Check sheet for the modelled part. Datum: model origin and axes. Units: mm. Round coordinates to 2 decimals unless told otherwise and drop trailing zeros. Loops run counter-clockwise (first coordinate to the right, second up) from the corner with the lowest first, then second, coordinate; pieces in that order, holes last. Notation, with made-up numbers: (-38, 25.5) - (7, 25.5) arc R14 ccw to (7, 43.5) - close; hole circle Ø8 at (50, -5.75). An arc over 180 degrees is marked (long way). Return JSON: item names as keys, results as strings.
Autodesk Inventor part; units mm, degrees
ref_plane "YZ Plane" through (0, 0, 0) normal (1, 0, 0) x (0, 1, 0)
ref_plane "XZ Plane" through (0, 0, 0) normal (0, 1, 0) x (-1, 0, 0)
ref_plane "XY Plane" through (0, 0, 0) normal (0, 0, 1) x (1, 0, 0)
sketch "Sketch1" plane through (0, 0, 0) normal (0, 0, 1) x (1, 0, 0)
  line L0 (350, -225) -> (-350, -225)
  line L1 (-335, 210) -> (335, 210)
  line L2 (335, 210) -> (335, -210)
  line L3 (335, -210) -> (-335, -210)
  line L4 (-335, -210) -> (-335, 210)
  line L5 (350, -225) -> (-350, -225)
  line L6 (350, 225) -> (350, -225)
  line L7 (-350, 225) -> (350, 225)
  line L8 (-350, -225) -> (-350, 225)
  line L9 (350, -210) -> (-350, -210)
  line L10 (-350, -225) -> (350, -225)
  point P0 (0, 0)
extrude "Extrusion1" add sketch "Sketch1" along normal blind 330.2 contours L0 L8 L9 L3 L6
sketch "Sketch2" plane through (-350, -210, 0) normal (0, 1, 0) x (1, 0, 0)
  line L0 (0, -330.2) -> (700, -330.2)
  line L1 (700, 0) -> (700, -330.2)
  line L2 (700, 0) -> (0, 0)
  line L3 (0, 0) -> (0, -330.2)
  line L4 (15, 0) -> (685, 0)
  line L5 (15, 0) -> (15, -330.2) construction
  line L6 (685, 0) -> (685, -330.2) construction
  line L7 (0, -12.7) -> (700, -12.7) construction
  line L8 (0, -317.5) -> (700, -317.5) construction
  line L9 (15, -12.7) -> (685, -12.7) construction
  line L10 (685, -12.7) -> (685, -317.5) construction
  line L11 (685, -317.5) -> (15, -317.5) construction
  line L12 (15, -317.5) -> (15, -12.7) construction
  line L13 (15, -317.5) -> (685, -317.5)
  line L14 (685, -317.5) -> (685, -12.7)
  line L15 (685, -12.7) -> (15, -12.7)
  line L16 (15, -12.7) -> (15, -317.5)
  point P0 (350, 0)
  dimension "d2" = 12.7
  dimension "d3" = 12.7
extrude "Extrusion2" cut sketch "Sketch2" against normal blind 4.7625 contours L16 L15 L14 L13
sketch "Sketch3" plane through (-350, -214.7625, 0) normal (0, 1, 0) x (1, 0, 0)
  line L0 (685, -12.7) -> (15, -12.7)
  line L1 (15, -12.7) -> (15, -317.5)
  line L2 (15, -317.5) -> (685, -317.5)
  line L3 (685, -317.5) -> (685, -12.7)
  line L4 (36.7157, -34.4157) -> (663.2843, -34.4157) construction
  line L5 (663.2843, -34.4157) -> (663.2843, -295.7843) construction
  line L6 (663.2843, -295.7843) -> (36.7157, -295.7843) construction
  line L7 (36.7157, -295.7843) -> (36.7157, -34.4157) construction
  circle A0 centre (36.7157, -34.4157) radius 5.1916
  circle A1 centre (663.2843, -34.4157) radius 5.1916
  circle A2 centre (663.2843, -295.7843) radius 5.1916
  circle A3 centre (36.7157, -295.7843) radius 5.1916
  point P0 (350, 0)
  dimension "d6" = 21.7157
  dimension "d7" = 10.3831
extrude "Extrusion3" add sketch "Sketch3" along normal blind 7.62 contours A0 | A1 | A2 | A3
fillet "Fillet1" radius 3.175 4 edges at (308.0927, -207.1425, 34.4157) (308.0927, -207.1425, 295.7843) (-318.4758, -207.1425, 295.7843) (-318.4758, -207.1425, 34.4157)
properties part number "BoxCover"
Q1. Sectioned sample at B-B (z = 226.5). Enter the section's corners in (x, y).
Answer key:
{"outline": "(-350, -225) - (350, -225) - (350, -210) - (335, -210) - (335, -214.76) - (-335, -214.76) - (-335, -210) - (-350, -210) - close"}
Q2. Depth check by flat-ended pin: P1, Ø12, axis at x = -15, z = 121.5, coming from the +Y side; P2, Ø2.5, axis at x = -158.5, y = -212.5, coming from the -Z side. Enter the tip coordinate at first touch or a pass-through.
Answer key:
{"P1": "stops at y = -214.76", "P2": "stops at z = 0"}
Q3. Sectioned sample at A-A (x = 84). Enter the section's corners in (y, z), plus the area to 3 significant figures.
Answer key:
{"outline": "(-225, 0) - (-210, 0) - (-210, 12.7) - (-214.76, 12.7) - (-214.76, 317.5) - (-210, 317.5) - (-210, 330.2) - (-225, 330.2) - close", "area": "3,500 mm²"}
Q4. Scan lines: probe 1 along Z at (x, y) = (272.5, -211.25); probe 2 along X at (y, z) = (-210.5, 98.5); probe 3 along Y at (x, z) = (16, 313.5). Record each from-to range of solid material in increasing order. Write a range as [from, to].
Answer key:
{"probe 1": "z = [0, 12.7], [317.5, 330.2]", "probe 2": "x = [-350, -335], [335, 350]", "probe 3": "y = [-225, -214.76]"}
Q5. Draft check along X on faces 1 (the face through (350, -217, 163)), 2 (the face through (-5, -217, 0)), 3 (the face through (-5, -214.762, 163)), 4 (the face through (-350, -218, 163)). Enter one of: released by +X, released by -X, zero draft, split by the parting line, or undercut.
Answer key:
{"face 1": "released by +X", "face 2": "zero draft", "face 3": "undercut", "face 4": "released by -X"}
